Design review of the part built by this model. Coordinates are the model's own, in mm. A direction names the side the tool comes from. Coordinates: 2 decimals unless noted, no trailing zeros. Write each loop counter-clockwise with the first axis right and the second up, starting at its lowest first coordinate (ties: lowest second). Pieces come first, ordered by that corner, then holes. Notation, with made-up numbers: (63, 9.5) - (72, 9.5) arc R21 ccw to (72, 39.5) - close; hole circle Ø9 at (-33.5, 63). An arc over 180 degrees is marked (long way). Answer as CSV lines item,"result". Start each with the question number.
Q1. Machinability: for faces 5 (the face through (14.252, 15.83, -30.827)), 6 (the face through (59.287, 0.507, -89.248)), 7 (the face through (50, 15, -31.54)), 8 (the face through (39.287, 0.493, -99.248)), 9 (the face through (86, 16, -11)), which of the approach directions +Z, -Z, +X, -X, +Y, -Y give a long, thin tool a straight path to every point of the face, cutting with its end or side? Answer none if there is none.
Q2. We need section D-D (z = -47.5). Write out the cut boundary in (x, y).
Q3. For line 1 along X through (y, z) = (15, -21); line 2 along Y through (x, z) = (72, -63.5); line 3 along Z through (x, y) = (35, 28), list the stretches that pass through material, from the lowest coordinate up. Write a range as [from, to].
Q4. Clearance check with flat-ended pins moving along their axes: pin 1 (3 mm diameter, centred on x = 44, y = 17, fed in from +Z); pin 2 (6 mm diameter, centred on x = 84.5, z = -36.5, fed in from +Y); pin 3 (10 mm diameter, centred on y = 13, z = -15, fed in from +X). State where each tip first meets the part, or that it passes through.
Q5. Mouldability with a two-part tool opening along Z and no side actions: class faces 1 (the face through (40.713, 0.507, -80.752)), 2 (the face through (49, 0, -51)), 3 (the face through (55.752, 0.507, -89.287)), 4 (the face through (50, 15, -10)) as pulls with the +Z half, pulls with the -Z half, needs draft (parallel to the pull), parting line crosses it, or undercut.
Q6. We need section A-A (y = 10). Write out the cut boundary in (x, z).
Q7. We need section C-C (z = -18). Write out the cut boundary in (x, y).
Q8. We need section B-B (x = 24). Write out the cut boundary in (y, z), plus the area to 3 significant figures.
from build123d import *

# Parameters (mm, degrees)
SKETCH2_W               = 100
SKETCH2_H               = 100
BOSS_EXTRUDE1_DEPTH     = 1
FILLET1_R               = 10
CUT_EXTRUDE1_DEPTH      = 142.424891727
CUT_EXTRUDE1_DEPTH_BACK = 142.424891727
FILLET2_R               = 2.5
SKETCH4_W               = 73
SKETCH4_H               = 21.54
BOSS_EXTRUDE2_DEPTH     = 29.32
FILLET3_R               = 2.5


with BuildPart() as part:
    # Sketch2 → Boss-Extrude1 (new body)
    with BuildSketch(Plane(origin=(0, 0, 0), x_dir=(1, 0, 0), z_dir=(0, 1, 0))):
        with Locations((50, 50)):
            Rectangle(SKETCH2_W, SKETCH2_H)
    extrude(amount=BOSS_EXTRUDE1_DEPTH)

    # Fillet1
    fillet1_edges = [part.edges().sort_by_distance(p)[0] for p in [
        (0, 0.5, -100),
        (100, 0.5, -100),
        (100, 0.5, 0),
        (0, 0.5, 0),
    ]]
    fillet(fillet1_edges, radius=FILLET1_R)

    # Sketch3 → Cut-Extrude1 (cut, two sides: drawn at the far end of the back side and taken through both)
    with BuildSketch(Plane(origin=(0, 1, 0), x_dir=(1, 0, 0), z_dir=(0, 1, 0)).offset(-CUT_EXTRUDE1_DEPTH_BACK)):
        Polygon((40, 343.238075794), (40, 100), (40, 80), (60, 80), (60, 90), (55, 90), (55, 85), (45, 85), (45, 100), (45, 343.238075794), (45, 829.714227381), (40, 829.714227381), align=None)
    extrude(amount=CUT_EXTRUDE1_DEPTH + CUT_EXTRUDE1_DEPTH_BACK, mode=Mode.SUBTRACT)

    # Fillet2
    fillet2_edges = [part.edges().sort_by_distance(p)[0] for p in [
        (60, 0.5, -80),
        (60, 0.5, -90),
        (55, 0.5, -90),
        (40, 0.5, -80),
    ]]
    fillet(fillet2_edges, radius=FILLET2_R - 0.0001)  # a hair under: the kernel refuses the full size
    fillet2_2_edges = [part.edges().sort_by_distance(p)[0] for p in [
        (45, 0.5, -100),
        (40, 0.5, -100),
        (55, 0.5, -85),
        (45, 0.5, -85),
    ]]
    fillet(fillet2_2_edges, radius=FILLET2_R)

    # Sketch4 → Boss-Extrude2 (add)
    with BuildSketch(Plane(origin=(0, 1, 0), x_dir=(1, 0, 0), z_dir=(0, 1, 0))):
        with Locations((50, 20.77)):
            Rectangle(SKETCH4_W, SKETCH4_H)
    extrude(amount=BOSS_EXTRUDE2_DEPTH)

    # Fillet3
    fillet3_edges = [part.edges().sort_by_distance(p)[0] for p in [
        (13.5, 1, -20.77),
        (13.5, 15.66, -31.54),
        (50, 1, -10),
        (13.5, 15.66, -10),
        (86.5, 1, -20.77),
        (86.5, 15.66, -10),
        (50, 1, -31.54),
        (86.5, 15.66, -31.54),
        (13.5, 30.32, -20.77),
        (50, 30.32, -10),
        (86.5, 30.32, -20.77),
        (50, 30.32, -31.54),
    ]]
    fillet(fillet3_edges, radius=FILLET3_R)


solid = part.part
Results list:
1,face 5,"-Z, -X, +Y"
1,face 6,"+Y, -Y"
1,face 7,"-Z, +X, -X, +Y"
1,face 8,"-Z, +Y, -Y"
1,face 9,"+Z, +X, +Y"
2,outline,"(0, 0) - (100, 0) - (100, 1) - (0, 1) - close"
3,line 1,"x = [13.5, 86.5]"
3,line 2,"y = [0, 1]"
3,line 3,"z = [-31.53, -10.01]"
4,pin 1,"stops at z = -10"
4,pin 2,"stops at y = 1.06"
4,pin 3,"stops at x = 86.5"
5,face 1,"pulls with the -Z half"
5,face 2,"needs draft"
5,face 3,"undercut"
5,face 4,"pulls with the +Z half"
6,outline,"(13.5, -29.04) arc R2.5 ccw to (16, -31.54) - (84, -31.54) arc R2.5 ccw to (86.5, -29.04) - (86.5, -12.5) arc R2.5 ccw to (84, -10) - (16, -10) arc R2.5 ccw to (13.5, -12.5) - close"
7,outline,"(0, 0) - (100, 0) - (100, 1) - (89, 1) arc R2.5 cw to (86.5, 3.5) - (86.5, 27.82) arc R2.5 ccw to (84, 30.32) - (16, 30.32) arc R2.5 ccw to (13.5, 27.82) - (13.5, 3.5) arc R2.5 cw to (11, 1) - (0, 1) - close"
8,outline,"(0, -100) - (1, -100) - (1, -34.04) arc R2.5 cw to (3.5, -31.54) - (27.82, -31.54) arc R2.5 ccw to (30.32, -29.04) - (30.32, -12.5) arc R2.5 ccw to (27.82, -10) - (3.5, -10) arc R2.5 cw to (1, -7.5) - (1, 0) - (0, 0) - close"
8,area,"732 mm2"
